The listing builds one solid part. Answer for the finished solid, in the listing's coordinates (mm). Give positions to 0.01 mm unless a question says otherwise; leave off trailing zeros.
Item 1: Consider line 1 along Y through (x, z) = (-6.5, -261); line 2 along Y through (x, z) = (14.5, -169.5); line 3 along X through (y, z) = (-6.25, 148.5). Determine where each line is inside the solid, lowest interval first.
Item 2: Each of these flat-tipped pins is pushed along its axis until it touches: pin 1 Ø0.8 at (x, z) = (-19, -50) entering from -Y; pin 2 Ø2.5 at (y, z) = (0.5, 71) entering from +X; pin 3 Ø2.5 at (x, z) = (-9.5, 17.5) entering from -Y. Where does it stop, or does it pass through?
Item 3: Section A-A, the plane z = -144.5 is taken. Give the number of separate pieces and of enclosed holes in the cut face, and give its area (4 significant figures).
from build123d import *

# Parameters (mm, degrees)
SKETCH1_R           = 2.1463
BOSS_EXTRUDE1_DEPTH = 457.2


with BuildPart() as part:
    # Sketch1 → Boss-Extrude1 (new body, symmetric)
    with BuildSketch(Plane.XY):
        with BuildLine():
            Line((-19.9898, 7.9883), (-19.9898, 3.2893))
            ThreePointArc((-19.9898, 3.2893), (-19.75917588, 2.73252412), (-19.2024, 2.5019))
            Line((-19.2024, 2.5019), (-18.4912, 2.5019))
            ThreePointArc((-18.4912, 2.5019), (-18.275673853, 2.591173853), (-18.1864, 2.8067))
            Line((-18.1864, 2.8067), (-18.1864, 4.9149))
            ThreePointArc((-18.1864, 4.9149), (-17.668965253, 5.689295824), (-16.755503096, 5.507596904))
            Line((-16.755503096, 5.507596904), (-14.500665747, 3.252759555))
            ThreePointArc((-14.500665747, 3.252759555), (-13.850954457, 2.280397894), (-13.622806192, 1.133419111))
            Line((-13.622806192, 1.133419111), (-13.622806192, -1.133419111))
            ThreePointArc((-13.622806192, -1.133419111), (-13.850954457, -2.280397894), (-14.500665747, -3.252759555))
            Line((-14.500665747, -3.252759555), (-16.755503096, -5.507596904))
            ThreePointArc((-16.755503096, -5.507596904), (-17.668965253, -5.689295824), (-18.1864, -4.9149))
            Line((-18.1864, -4.9149), (-18.1864, -2.8067))
            ThreePointArc((-18.1864, -2.8067), (-18.275673853, -2.591173853), (-18.4912, -2.5019))
            Line((-18.4912, -2.5019), (-19.2024, -2.5019))
            ThreePointArc((-19.2024, -2.5019), (-19.75917588, -2.73252412), (-19.9898, -3.2893))
            Line((-19.9898, -3.2893), (-19.9898, -7.9883))
            ThreePointArc((-19.9898, -7.9883), (-19.402080467, -9.407180467), (-17.9832, -9.9949))
            Line((-17.9832, -9.9949), (-13.2842, -9.9949))
            ThreePointArc((-13.2842, -9.9949), (-12.72742412, -9.76427588), (-12.4968, -9.2075))
            Line((-12.4968, -9.2075), (-12.4968, -8.4963))
            ThreePointArc((-12.4968, -8.4963), (-12.586073853, -8.280773853), (-12.8016, -8.1915))
            Line((-12.8016, -8.1915), (-14.9098, -8.1915))
            ThreePointArc((-14.9098, -8.1915), (-15.684195824, -7.674065253), (-15.502496904, -6.760603096))
            Line((-15.502496904, -6.760603096), (-13.247659555, -4.505765747))
            ThreePointArc((-13.247659555, -4.505765747), (-12.275297894, -3.856054457), (-11.128319111, -3.627906192))
            Line((-11.128319111, -3.627906192), (-8.861480889, -3.627906192))
            ThreePointArc((-8.861480889, -3.627906192), (-7.714502106, -3.856054457), (-6.742140445, -4.505765747))
            Line((-6.742140445, -4.505765747), (-4.487303096, -6.760603096))
            ThreePointArc((-4.487303096, -6.760603096), (-4.305604176, -7.674065253), (-5.08, -8.1915))
            Line((-5.08, -8.1915), (-7.1882, -8.1915))
            ThreePointArc((-7.1882, -8.1915), (-7.403726147, -8.280773853), (-7.493, -8.4963))
            Line((-7.493, -8.4963), (-7.493, -9.2075))
            ThreePointArc((-7.493, -9.2075), (-7.26237588, -9.76427588), (-6.7056, -9.9949))
            Line((-6.7056, -9.9949), (0, -9.9949))
            Line((0, -9.9949), (6.7056, -9.9949))
            ThreePointArc((6.7056, -9.9949), (7.26237588, -9.76427588), (7.493, -9.2075))
            Line((7.493, -9.2075), (7.493, -8.4963))
            ThreePointArc((7.493, -8.4963), (7.403726147, -8.280773853), (7.1882, -8.1915))
            Line((7.1882, -8.1915), (5.08, -8.1915))
            ThreePointArc((5.08, -8.1915), (4.305604176, -7.674065253), (4.487303096, -6.760603096))
            Line((4.487303096, -6.760603096), (6.742140445, -4.505765747))
            ThreePointArc((6.742140445, -4.505765747), (7.714502106, -3.856054457), (8.861480889, -3.627906192))
            Line((8.861480889, -3.627906192), (11.128319111, -3.627906192))
            ThreePointArc((11.128319111, -3.627906192), (12.275297894, -3.856054457), (13.247659555, -4.505765747))
            Line((13.247659555, -4.505765747), (15.502496904, -6.760603096))
            ThreePointArc((15.502496904, -6.760603096), (15.684195824, -7.674065253), (14.9098, -8.1915))
            Line((14.9098, -8.1915), (12.8016, -8.1915))
            ThreePointArc((12.8016, -8.1915), (12.586073853, -8.280773853), (12.4968, -8.4963))
            Line((12.4968, -8.4963), (12.4968, -9.2075))
            ThreePointArc((12.4968, -9.2075), (12.72742412, -9.76427588), (13.2842, -9.9949))
            Line((13.2842, -9.9949), (17.9832, -9.9949))
            ThreePointArc((17.9832, -9.9949), (19.402080467, -9.407180467), (19.9898, -7.9883))
            Line((19.9898, -7.9883), (19.9898, -3.2893))
            ThreePointArc((19.9898, -3.2893), (19.75917588, -2.73252412), (19.2024, -2.5019))
            Line((19.2024, -2.5019), (18.4912, -2.5019))
            ThreePointArc((18.4912, -2.5019), (18.275673853, -2.591173853), (18.1864, -2.8067))
            Line((18.1864, -2.8067), (18.1864, -4.9149))
            ThreePointArc((18.1864, -4.9149), (17.668965253, -5.689295824), (16.755503096, -5.507596904))
            Line((16.755503096, -5.507596904), (14.500665747, -3.252759555))
            ThreePointArc((14.500665747, -3.252759555), (13.850954457, -2.280397894), (13.622806192, -1.133419111))
            Line((13.622806192, -1.133419111), (13.622806192, 1.133419111))
            ThreePointArc((13.622806192, 1.133419111), (13.850954457, 2.280397894), (14.500665747, 3.252759555))
            Line((14.500665747, 3.252759555), (16.755503096, 5.507596904))
            ThreePointArc((16.755503096, 5.507596904), (17.668965253, 5.689295824), (18.1864, 4.9149))
            Line((18.1864, 4.9149), (18.1864, 2.8067))
            ThreePointArc((18.1864, 2.8067), (18.275673853, 2.591173853), (18.4912, 2.5019))
            Line((18.4912, 2.5019), (19.2024, 2.5019))
            ThreePointArc((19.2024, 2.5019), (19.75917588, 2.73252412), (19.9898, 3.2893))
            Line((19.9898, 3.2893), (19.9898, 7.9883))
            ThreePointArc((19.9898, 7.9883), (19.402080467, 9.407180467), (17.9832, 9.9949))
            Line((17.9832, 9.9949), (13.2842, 9.9949))
            ThreePointArc((13.2842, 9.9949), (12.72742412, 9.76427588), (12.4968, 9.2075))
            Line((12.4968, 9.2075), (12.4968, 8.4963))
            ThreePointArc((12.4968, 8.4963), (12.586073853, 8.280773853), (12.8016, 8.1915))
            Line((12.8016, 8.1915), (14.9098, 8.1915))
            ThreePointArc((14.9098, 8.1915), (15.684195824, 7.674065253), (15.502496904, 6.760603096))
            Line((15.502496904, 6.760603096), (13.247659555, 4.505765747))
            ThreePointArc((13.247659555, 4.505765747), (12.275297894, 3.856054457), (11.128319111, 3.627906192))
            Line((11.128319111, 3.627906192), (8.861480889, 3.627906192))
            ThreePointArc((8.861480889, 3.627906192), (7.714502106, 3.856054457), (6.742140445, 4.505765747))
            Line((6.742140445, 4.505765747), (4.487303096, 6.760603096))
            ThreePointArc((4.487303096, 6.760603096), (4.305604176, 7.674065253), (5.08, 8.1915))
            Line((5.08, 8.1915), (7.1882, 8.1915))
            ThreePointArc((7.1882, 8.1915), (7.403726147, 8.280773853), (7.493, 8.4963))
            Line((7.493, 8.4963), (7.493, 9.2075))
            ThreePointArc((7.493, 9.2075), (7.26237588, 9.76427588), (6.7056, 9.9949))
            Line((6.7056, 9.9949), (0, 9.9949))
            Line((0, 9.9949), (-6.7056, 9.9949))
            ThreePointArc((-6.7056, 9.9949), (-7.26237588, 9.76427588), (-7.493, 9.2075))
            Line((-7.493, 9.2075), (-7.493, 8.4963))
            ThreePointArc((-7.493, 8.4963), (-7.403726147, 8.280773853), (-7.1882, 8.1915))
            Line((-7.1882, 8.1915), (-5.08, 8.1915))
            ThreePointArc((-5.08, 8.1915), (-4.305604176, 7.674065253), (-4.487303096, 6.760603096))
            Line((-4.487303096, 6.760603096), (-6.742140445, 4.505765747))
            ThreePointArc((-6.742140445, 4.505765747), (-7.714502106, 3.856054457), (-8.861480889, 3.627906192))
            Line((-8.861480889, 3.627906192), (-11.128319111, 3.627906192))
            ThreePointArc((-11.128319111, 3.627906192), (-12.275297894, 3.856054457), (-13.247659555, 4.505765747))
            Line((-13.247659555, 4.505765747), (-15.502496904, 6.760603096))
            ThreePointArc((-15.502496904, 6.760603096), (-15.684195824, 7.674065253), (-14.9098, 8.1915))
            Line((-14.9098, 8.1915), (-12.8016, 8.1915))
            ThreePointArc((-12.8016, 8.1915), (-12.586073853, 8.280773853), (-12.4968, 8.4963))
            Line((-12.4968, 8.4963), (-12.4968, 9.2075))
            ThreePointArc((-12.4968, 9.2075), (-12.72742412, 9.76427588), (-13.2842, 9.9949))
            Line((-13.2842, 9.9949), (-17.9832, 9.9949))
            ThreePointArc((-17.9832, 9.9949), (-19.402080467, 9.407180467), (-19.9898, 7.9883))
        make_face()
        with Locations((-9.9949, 0)):
            Circle(SKETCH1_R, mode=Mode.SUBTRACT)
        with Locations((9.9949, 0)):
            Circle(SKETCH1_R, mode=Mode.SUBTRACT)
        with BuildLine():
            Line((-6.366993808, 1.133419111), (-6.366993808, -1.133419111))
            ThreePointArc((-6.366993808, -1.133419111), (-6.138845543, -2.280397894), (-5.489134253, -3.252759555))
            Line((-5.489134253, -3.252759555), (-0.939581002, -7.802312806))
            ThreePointArc((-0.939581002, -7.802312806), (0, -8.1915), (0.939581002, -7.802312806))
            Line((0.939581002, -7.802312806), (5.489134253, -3.252759555))
            ThreePointArc((5.489134253, -3.252759555), (6.138845543, -2.280397894), (6.366993808, -1.133419111))
            Line((6.366993808, -1.133419111), (6.366993808, 1.133419111))
            ThreePointArc((6.366993808, 1.133419111), (6.138845543, 2.280397894), (5.489134253, 3.252759555))
            Line((5.489134253, 3.252759555), (0.939581002, 7.802312806))
            ThreePointArc((0.939581002, 7.802312806), (0, 8.1915), (-0.939581002, 7.802312806))
            Line((-0.939581002, 7.802312806), (-5.489134253, 3.252759555))
            ThreePointArc((-5.489134253, 3.252759555), (-6.138845543, 2.280397894), (-6.366993808, 1.133419111))
        make_face(mode=Mode.SUBTRACT)
    extrude(amount=BOSS_EXTRUDE1_DEPTH, both=True)


solid = part.part
Worked answers:
1. line 1: y = -9.99 to -8.19, -4.75 to 4.75, 8.19 to 9.99
1. line 2: y = -9.99 to -8.19, -5.76 to -3.25, 3.25 to 5.76, 8.19 to 9.99
1. line 3: x = -19.99 to -14.99, -5 to -2.49, 2.49 to 5, 14.99 to 19.99
2. pin 1: stops at y = -9.9
2. pin 2: stops at x = 13.69
2. pin 3: stops at y = -3.69
3. separate pieces: 1
3. enclosed holes: 3
3. area: 328.5 mm2
